Geometry check sheet. Reference: the model listing, model coordinates, mm. Face numbers are marked on the shaded views. A direction names the side the tool comes from. Give positions to 0.01 mm unless a question says otherwise; leave off trailing zeros. Write each loop counter-clockwise with the first axis right and the second up, starting at its lowest first coordinate (ties: lowest second). Pieces come first, ordered by that corner, then holes. Notation, with made-up numbers: (60.25, 12) -> (112.25, 12) arc R26 ccw to (112.25, 27) -> close; hole circle Ø10 at (-18.5, 74). An arc over 180 degrees is marked (long way). One line per item, written item: value.
from build123d import *

# Parameters (mm, degrees)
SKETCH_1_W      = 12
SKETCH_1_H      = 6
SKETCH_1_W_2    = 6
SKETCH_1_H_2    = 3
EXTRUDE_1_DEPTH = 5
SKETCH_2_W      = 11.46002803
SKETCH_2_H      = 5.61022278
SKETCH_2_W_2    = 1.5
SKETCH_2_H_2    = 0.606360044
EXTRUDE_2_DEPTH = 0.5
SKETCH_2_3_W    = 0.269985985
SKETCH_2_3_H    = 5.61022278
EXTRUDE_3_DEPTH = 1.5
SKETCH_2_4_W    = 0.980014015
SKETCH_2_4_H    = 0.606360044
SKETCH_2_4_W_2  = 0.519985985
SKETCH_2_4_W_3  = 1.5
EXTRUDE_4_DEPTH = 4
SKETCH_4_W      = 6
SKETCH_4_H      = 3
EXTRUDE_5_DEPTH = 4.5
SKETCH_6_W      = 3
SKETCH_6_H      = 3
EXTRUDE_6_DEPTH = 5.5


with BuildPart() as part:
    # Sketch 1 → Extrude 1 (new body)
    with BuildSketch(Plane(origin=(0, 0, 0), x_dir=(1, 0, 0), z_dir=(0, 1, 0))):
        Rectangle(SKETCH_1_W, SKETCH_1_H)
        Rectangle(SKETCH_1_W_2, SKETCH_1_H_2, mode=Mode.SUBTRACT)
    extrude(amount=EXTRUDE_1_DEPTH)

    # Sketch 2 → Extrude 2 (add)
    with BuildSketch(Plane(origin=(0, 5, 0), x_dir=(1, 0, 0), z_dir=(0, 1, 0))):
        Rectangle(SKETCH_2_W, SKETCH_2_H)
        Polygon((3.980014015, -0.303180022), (3, -0.303180022), (3, -1.5), (-3, -1.5), (-3, -0.303180022), (-3.980014015, -0.303180022), (-3.980014015, 0.303180022), (-3, 0.303180022), (-3, 1.5), (3, 1.5), (3, 0.303180022), (3.980014015, 0.303180022), align=None, mode=Mode.SUBTRACT)
        Polygon((3, -0.303180022), (2.480014015, -0.303180022), (2.480014015, 0.303180022), (3, 0.303180022), (3, 1.5), (-3, 1.5), (-3, 0.303180022), (-2.480014015, 0.303180022), (-2.480014015, -0.303180022), (-3, -0.303180022), (-3, -1.5), (3, -1.5), align=None)
        Rectangle(SKETCH_2_W_2, SKETCH_2_H_2, mode=Mode.SUBTRACT)
    extrude(amount=EXTRUDE_2_DEPTH)

    # Sketch 2_3 → Extrude 3 (add)
    with BuildSketch(Plane(origin=(0, 5, 0), x_dir=(1, 0, 0), z_dir=(0, 1, 0))):
        with Locations((-5.865007008, 0)):
            Rectangle(SKETCH_2_3_W, SKETCH_2_3_H)
        with Locations((5.865007008, 0)):
            Rectangle(SKETCH_2_3_W, SKETCH_2_3_H)
    extrude(amount=EXTRUDE_3_DEPTH)

    # Sketch 2_4 → Extrude 4 (add)
    with BuildSketch(Plane(origin=(0, 5, 0), x_dir=(1, 0, 0), z_dir=(0, 1, 0))):
        with Locations((3.490007008, 0)):
            Rectangle(SKETCH_2_4_W, SKETCH_2_4_H)
        with Locations((2.740007008, 0)):
            Rectangle(SKETCH_2_4_W_2, SKETCH_2_4_H)
        Rectangle(SKETCH_2_4_W_3, SKETCH_2_4_H)
        with Locations((-2.740007008, 0)):
            Rectangle(SKETCH_2_4_W_2, SKETCH_2_4_H)
        with Locations((-3.490007008, 0)):
            Rectangle(SKETCH_2_4_W, SKETCH_2_4_H)
    extrude(amount=EXTRUDE_4_DEPTH)

    # Sketch 4 → Extrude 5 (add)
    with BuildSketch(Plane.XZ.offset(-5)):
        Rectangle(SKETCH_4_W, SKETCH_4_H)
    extrude(amount=EXTRUDE_5_DEPTH)

    # Sketch 6 → Extrude 6 (add)
    with BuildSketch(Plane.XZ.offset(-0.5)):
        with Locations((1.5, 0)):
            Rectangle(SKETCH_6_W, SKETCH_6_H)
    extrude(amount=EXTRUDE_6_DEPTH)


solid = part.part
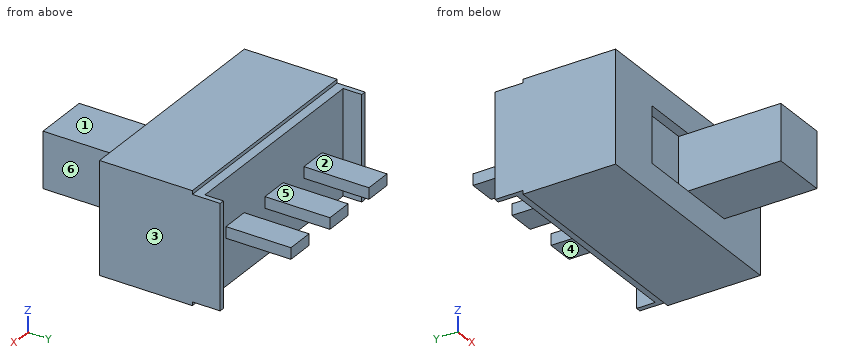
1) Scan lines: probe 1 along X at (y, z) = (6.25, -1.55); probe 2 along Y at (x, z) = (-1, 0.5); probe 3 along Z at (x, y) = (2, -4.5). Record each from-to range of solid material in increasing order.
Verdict:
probe 1: -6 to -5.73, 5.73 to 6
probe 2: 0.5 to 5.5
probe 3: -1.5 to 1.5
2) Sectioned sample at A-A on y = 7. Record the cut outline in (x, z).
Verdict:
outline: (-3.98, -0.3) -> (-2.48, -0.3) -> (-2.48, 0.3) -> (-3.98, 0.3) -> close; (-0.75, -0.3) -> (0.75, -0.3) -> (0.75, 0.3) -> (-0.75, 0.3) -> close; (2.48, -0.3) -> (3.98, -0.3) -> (3.98, 0.3) -> (2.48, 0.3) -> close
3) Sectioned sample at D-D on y = -2.75. Record the cut outline in (x, z), plus the area to 3 significant figures.
Verdict:
outline: (0, -1.5) -> (3, -1.5) -> (3, 1.5) -> (0, 1.5) -> close
area: 9.00 mm^2
4) Sectioned sample at C-C on x = 0.25. Record the cut outline in (y, z), plus the area to 3 significant figures.
Verdict:
outline: (-5, -1.5) -> (0, -1.5) -> (0, -3) -> (5, -3) -> (5, -2.81) -> (5.5, -2.81) -> (5.5, -0.3) -> (9, -0.3) -> (9, 0.3) -> (5.5, 0.3) -> (5.5, 2.81) -> (5, 2.81) -> (5, 3) -> (0, 3) -> (0, 1.5) -> (-5, 1.5) -> close
area: 49.9 mm^2
5) Mould release check, pull along X, two halves, no side actions. Record for the marked faces 1, 2 and 3: released by +X, released by -X, zero draft, split by the parting line, or undercut.
Verdict:
face 1: zero draft
face 2: undercut
face 3: released by +X
6) Depth check by flat-ended pin: pin 1 Ø0.8 at (x, y) = (3, 7.5) entering from +Z; pin 2 Ø1.5 at (x, y) = (1.5, -3.5) entering from -Z; pin 3 Ø0.8 at (x, y) = (2.5, 6) entering from -Z. Enter the tip coordinate at first touch or a pass-through.
Verdict:
pin 1: z = 0.3
pin 2: z = -1.5
pin 3: z = -0.3
7) Tool access check on the marked faces 4, 5 and 6. Record the directions out of +Z, -Z, +X, -X, +Y, -Y that give a thin tool (end or side, any length) a straight path to the whole face; none if there is none.
Verdict:
face 4: -Z, +Y
face 5: +Z, +Y
face 6: +Z, -Z, +X, -Y
8) Sectioned sample at B-B on z = -1.05. Record the cut outline in (x, y).
Verdict:
outline: (-6, 0) -> (-3, 0) -> (-3, 0.5) -> (0, 0.5) -> (0, -5) -> (3, -5) -> (3, 0) -> (6, 0) -> (6, 6.5) -> (5.73, 6.5) -> (5.73, 5.5) -> (-5.73, 5.5) -> (-5.73, 6.5) -> (-6, 6.5) -> close
